```python
from build123d import *

# Parameters (mm, degrees)
SKETCH2_R           = 5.5
BOSS_EXTRUDE1_DEPTH = 8
SKETCH6_W           = 82
SKETCH6_H           = 72
BOSS_EXTRUDE4_DEPTH = 45
BOSS_EXTRUDE5_DEPTH = 5
CUT_EXTRUDE1_DEPTH  = 35
FILLET1_R           = 6
SKETCH9_R           = 15
SKETCH9_R_2         = 3
CUT_EXTRUDE2_DEPTH  = 98.775252493
RIB2_REACH          = 99.775
SKETCH11_WALL_W     = 251.085540362
SKETCH11_WALL_H     = 10


with BuildPart() as part:
    # Sketch2 → Boss-Extrude1 (new body)
    with BuildSketch(Plane(origin=(0, 0, 0), x_dir=(1, 0, 0), z_dir=(0, 1, 0))):
        with BuildLine():
            Line((-59, -36), (59, -36))
            ThreePointArc((59, -36), (66.778174593, -32.778174593), (70, -25))
            Line((70, -25), (70, 25))
            ThreePointArc((70, 25), (66.778174593, 32.778174593), (59, 36))
            Line((59, 36), (-59, 36))
            ThreePointArc((-59, 36), (-66.778174593, 32.778174593), (-70, 25))
            Line((-70, 25), (-70, -25))
            ThreePointArc((-70, -25), (-66.778174593, -32.778174593), (-59, -36))
        make_face()
        with Locations(Location((-56, 25, 0), (0, 0, 270))):
            Circle(SKETCH2_R, mode=Mode.SUBTRACT)
        with Locations(Location((-56, -25, 0), (0, 0, 270))):
            Circle(SKETCH2_R, mode=Mode.SUBTRACT)
        with Locations(Location((56, 25, 0), (0, 0, 270))):
            Circle(SKETCH2_R, mode=Mode.SUBTRACT)
        with Locations(Location((56, -25, 0), (0, 0, 270))):
            Circle(SKETCH2_R, mode=Mode.SUBTRACT)
    extrude(amount=BOSS_EXTRUDE1_DEPTH)

    # Sketch6 → Boss-Extrude4 (add)
    with BuildSketch(Plane(origin=(0, 8, 0), x_dir=(1, 0, 0), z_dir=(0, 1, 0))):
        Rectangle(SKETCH6_W, SKETCH6_H)
    extrude(amount=BOSS_EXTRUDE4_DEPTH)

    # Sketch7 → Boss-Extrude5 (add)
    with BuildSketch(Plane(origin=(0, 53, 0), x_dir=(1, 0, 0), z_dir=(0, 1, 0))):
        with BuildLine():
            ThreePointArc((-16.25, -11.659223816), (0, -20), (16.25, -11.659223816))
            ThreePointArc((16.25, -11.659223816), (19.968227615, -8.512179491), (24.732142857, -7.495215311))
            ThreePointArc((24.732142857, -7.495215311), (32.5, 0), (24.732142857, 7.495215311))
            ThreePointArc((24.732142857, 7.495215311), (19.968227615, 8.512179491), (16.25, 11.659223816))
            ThreePointArc((16.25, 11.659223816), (0, 20), (-16.25, 11.659223816))
            ThreePointArc((-16.25, 11.659223816), (-19.968227615, 8.512179491), (-24.732142857, 7.495215311))
            ThreePointArc((-24.732142857, 7.495215311), (-32.5, 0), (-24.732142857, -7.495215311))
            ThreePointArc((-24.732142857, -7.495215311), (-19.968227615, -8.512179491), (-16.25, -11.659223816))
        make_face()
    extrude(amount=BOSS_EXTRUDE5_DEPTH)

    # Sketch8 → Cut-Extrude1 (cut)
    with BuildSketch(Plane.XZ):
        with BuildLine():
            Line((-26.5, -31.5), (26.5, -31.5))
            ThreePointArc((26.5, -31.5), (30.742640687, -29.742640687), (32.5, -25.5))
            Line((32.5, -25.5), (32.5, 25.5))
            ThreePointArc((32.5, 25.5), (30.742640687, 29.742640687), (26.5, 31.5))
            Line((26.5, 31.5), (-26.5, 31.5))
            ThreePointArc((-26.5, 31.5), (-30.742640687, 29.742640687), (-32.5, 25.5))
            Line((-32.5, 25.5), (-32.5, -25.5))
            ThreePointArc((-32.5, -25.5), (-30.742640687, -29.742640687), (-26.5, -31.5))
        make_face()
    extrude(amount=-CUT_EXTRUDE1_DEPTH, mode=Mode.SUBTRACT)

    # Fillet1
    fillet1_edges = [part.edges().sort_by_distance(p)[0] for p in [
        (-30.742640687, 35, -29.742640687),
        (-32.5, 35, 0),
        (-30.742640687, 35, 29.742640687),
        (0, 35, 31.5),
        (30.742640687, 35, 29.742640687),
        (32.5, 35, 0),
        (30.742640687, 35, -29.742640687),
        (0, 35, -31.5),
    ]]
    fillet(fillet1_edges, radius=FILLET1_R)

    # Sketch9 → Cut-Extrude2 (cut, through all)
    with BuildSketch(Plane(origin=(0, 58, 0), x_dir=(1, 0, 0), z_dir=(0, 1, 0))):
        with Locations(Location((0, 0, 0), (0, 0, 270))):
            Circle(SKETCH9_R)
        with Locations(Location((25, 0, 0), (0, 0, 270))):
            Circle(SKETCH9_R_2)
        with Locations(Location((-25, 0, 0), (0, 0, 270))):
            Circle(SKETCH9_R_2)
    extrude(amount=-CUT_EXTRUDE2_DEPTH, mode=Mode.SUBTRACT)

    # Sketch11 wall → Rib2 (add, up to next)
    with BuildSketch(Plane(origin=(-55.5, 30.5, 0), x_dir=(-0.541701333727, -0.840571035094, 0), z_dir=(0.840571035094, -0.541701333727, 0)), mode=Mode.PRIVATE) as rib2_sk1:
        Rectangle(SKETCH11_WALL_W, SKETCH11_WALL_H)
    rib2_tool1 = extrude(rib2_sk1.sketch, amount=RIB2_REACH, mode=Mode.PRIVATE) - part.part
    rib2 = rib2_tool1.solids().sort_by_distance((-55.5, 30.5, 0))[0]
    add(rib2)

    # Mirror1: Rib2 across plane
    add(rib2.mirror(Plane(origin=(0, 0, 0), x_dir=(0, 0, 1), z_dir=(1, 0, 0))))


solid = part.part
```
The listing builds one solid part. Answer for the finished solid, in the listing's coordinates (mm). A direction names the side the tool comes from. Round coordinates to 2 decimals unless told otherwise and drop trailing zeros. Order: outer loops, then holes, each group sorted by start corner. A loop starts at its lowest first (then second) coordinate and runs counter-clockwise, first axis right, second up. Notation, with made-up numbers: (0, -32.5) - (12, -32.5) arc R19 cw to (12, -12.5) - close; hole circle Ø7 at (28.25, -8). An arc over 180 degrees is marked (long way). Put each result on its own line as item: value. Start each with the question number.
(1) Find section D-D (z = -10). Give the vertices of the cut face in (x, y), plus the area to 3 significant figures.
(2) Find section C-C (y = 46). Give the vertices of the cut face in (x, z).
(3) For faces 4 (the flat face through (51, 21, -5)), 5 (the flat face through (-1, 53, -25)), 6 (the flat face through (51, 21, 5)), determine the directions among +Z, -Z, +X, -X, +Y, -Y from which every point of the face is accessible in a straight line to the end or side of a thin tool.
(4) Determine the mould class of faces 1 (the flat face through (-51, 21, -5)), 2 (the flat face through (-10, 58, 12)), 3 (the cylindrical face through (-30.696, 14.297, 29.789)) for opening direction Z: released by +Z, released by -Z, zero draft, split by the parting line, or undercut.
(5) Straight lines are drawn through the part: probe 1 along X at (y, z) = (5, -25); probe 2 along X at (y, z) = (22.5, 8.5); probe 3 along X at (y, z) = (40, 0). For each, find the intervals that lie inside material, in ascending order. Write a range as from..to.
(6) Find section A-A (z = 0). Give the vertices of the cut face in (x, y), plus the area to 3 significant figures.
(7) Given P1, Ø9, axis at x = -56, z = -25, coming from the +Y side; P2, Ø8.5, axis at x = -57, z = 27, coming from the +Y side; P3, Ø4, axis at y = 35, z = 22, coming from the +X side; P4, Ø5, axis at y = 12, z = -28, coming from the -X side, each flat-ended and moving along its own axis, determine where each tip first touches the part or whether it passes through.
(8) Find section B-B (x = 7.5). Give the vertices of the cut face in (y, z).
Reply:
1. outline: (-70, 0) - (-32.5, 0) - (-32.5, 29) arc R6 cw to (-26.5, 35) - (-11.18, 35) - (-11.18, 58) - (-17.75, 58) - (-17.75, 53) - (-41, 53) - (-41, 8) - (-70, 8) - close; (11.18, 35) - (26.5, 35) arc R6 cw to (32.5, 29) - (32.5, 0) - (70, 0) - (70, 8) - (41, 8) - (41, 53) - (17.75, 53) - (17.75, 58) - (11.18, 58) - close
1. area: 2,210 mm^2
2. outline: (-45.51, -5) - (-41, -5) - (-41, -36) - (41, -36) - (41, -5) - (45.51, -5) - (45.51, 5) - (41, 5) - (41, 36) - (-41, 36) - (-41, 5) - (-45.51, 5) - close; hole circle Ø6 at (-25, 0); hole circle Ø30 at (0, 0); hole circle Ø6 at (25, 0)
3. face 4: -Z, +X, +Y
3. face 5: +Y
3. face 6: +Z, +X, +Y
4. face 1: released by -Z
4. face 2: zero draft
4. face 3: undercut
5. probe 1: -70..-61.5, -50.5..-32.5, 32.5..50.5, 61.5..70
5. probe 2: -41..-32.5, 32.5..41
5. probe 3: -49.38..-28, -22..-15, 15..22, 28..49.38
6. outline: (-70, 0) - (-32.5, 0) - (-32.5, 29) arc R6 cw to (-28, 34.81) - (-28, 58) - (-32.5, 58) - (-32.5, 53) - (-41, 53) - (-70, 8) - close; (-22, 35) - (-15, 35) - (-15, 58) - (-22, 58) - close; (15, 35) - (22, 35) - (22, 58) - (15, 58) - close; (28, 34.81) arc R6 cw to (32.5, 29) - (32.5, 0) - (70, 0) - (70, 8) - (41, 53) - (32.5, 53) - (32.5, 58) - (28, 58) - close
6. area: 3,210 mm^2
7. P1: through
7. P2: y = 8
7. P3: x = 41
7. P4: x = -41
8. outline: (0, -36) - (53, -36) - (53, -18.54) - (58, -18.54) - (58, -12.99) - (35, -12.99) - (35, -25.5) arc R6 cw to (29, -31.5) - (0, -31.5) - close; (0, 31.5) - (29, 31.5) arc R6 cw to (35, 25.5) - (35, 12.99) - (58, 12.99) - (58, 18.54) - (53, 18.54) - (53, 36) - (0, 36) - close
